Part print with two shaded views. Sizes in mm from the minimum x, y, z corner. A direction names the side the tool comes from. Coordinates: 2 decimals unless noted, no trailing zeros. Order: outer loops, then holes, each group sorted by start corner. A loop starts at its lowest first (then second) coordinate and runs counter-clockwise, first axis right, second up. Notation, with made-up numbers: M 33,49.5 L 53,49.5 A29 cw 53,88.5 Z; hole C -4,21.25 d5. An arc over 180 degrees is marked long. Answer in a Markdown table with one row per item. Add a question column.
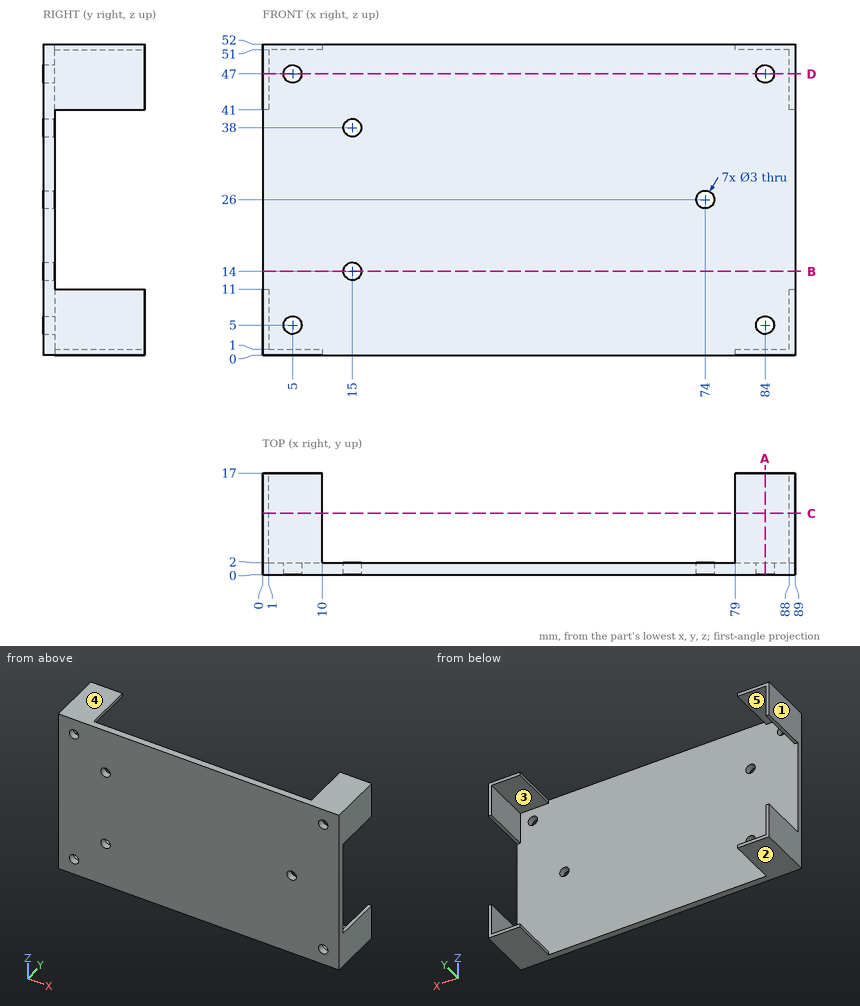
(1) Slice it at B-B (z = 14). List the corners of the cut face in (x, y).
(2) Slice it at C-C (y = 10.25). List the corners of the cut face in (x, z), and give its area (3 significant figures).
(3) Slice it at D-D (z = 47). List the corners of the cut face in (x, y), and give its area (3 significant figures).
(4) 3-axis set-ups, long thin cutter, end or side, ignore diameter. For the marked faces 4 and 5: which of +Z, -Z, +X, -X, +Y, -Y reach the whole face in a straight line?
(5) Drop a flat-ended pin along its axis: P1, Ø5, axis at x = 84, z = 47, coming from the +Y side. Give the stop position or say it passes through.
(6) Pull direction X, two halves, no side cores. Call the marked faces 1, 2 and 3: pulls with the +X half, pulls with the -X half, needs draft (parallel to the pull), parting line crosses it, or undercut.
(7) Wall check: line 1 (Z direction, x = 5, y = 0.55); line 2 (X direction, y = 9.5, z = 43); line 3 (X direction, y = 0.55, z = 47). Give the ranges that are in metal, low to high.
(8) Slice it at A-A (x = 84). List the corners of the cut face in (y, z).
Computed:
| question | item | result |
|---|---|---|
| 1 | outline | M 0,0 L 13.5,0 L 13.5,2 L 0,2 Z; M 16.5,0 L 89,0 L 89,2 L 16.5,2 Z |
| 2 | outline | M 0,0 L 10,0 L 10,1 L 1,1 L 1,11 L 0,11 Z; M 0,41 L 1,41 L 1,51 L 10,51 L 10,52 L 0,52 Z; M 79,0 L 89,0 L 89,11 L 88,11 L 88,1 L 79,1 Z; M 79,51 L 88,51 L 88,41 L 89,41 L 89,52 L 79,52 Z |
| 2 | area | 80.0 mm^2 |
| 3 | outline | M 0,0 L 3.5,0 L 3.5,2 L 1,2 L 1,17 L 0,17 Z; M 6.5,0 L 82.5,0 L 82.5,2 L 6.5,2 Z; M 85.5,0 L 89,0 L 89,17 L 88,17 L 88,2 L 85.5,2 Z |
| 3 | area | 196 mm^2 |
| 4 | face 4 | +Z, +X, -X, +Y, -Y |
| 4 | face 5 | +Y |
| 5 | P1 | stops at y = 2 |
| 6 | face 1 | pulls with the -X half |
| 6 | face 2 | needs draft |
| 6 | face 3 | undercut |
| 7 | line 1 | z = 0 to 3.5, 6.5 to 45.5, 48.5 to 52 |
| 7 | line 2 | x = 0 to 1, 88 to 89 |
| 7 | line 3 | x = 0 to 3.5, 6.5 to 82.5, 85.5 to 89 |
| 8 | outline | M 0,0 L 17,0 L 17,1 L 2,1 L 2,3.5 L 0,3.5 Z; M 0,6.5 L 2,6.5 L 2,45.5 L 0,45.5 Z; M 0,48.5 L 2,48.5 L 2,51 L 17,51 L 17,52 L 0,52 Z |
